Source: CAD feature listing. Evaluate the final solid. Frame: model axes, mm. A direction names the side the tool comes from. Round coordinates to 2 decimals unless told otherwise and drop trailing zeros. Write each loop counter-clockwise with the first axis right and the second up, starting at its lowest first coordinate (ties: lowest second). Pieces come first, ordered by that corner, then holes. Notation, with made-up numbers: M -28.75,-19.75 L 16.25,-19.75 A19 cw 16.25,-10.75 Z; hole C 75,-21 d3. An arc over 180 degrees is marked long. Answer in a Markdown table with one row per item.
from build123d import *

# Parameters (mm, degrees)
SKETCH1_W           = 2.4
SKETCH1_H           = 100
SKETCH1_W_2         = 92
SKETCH1_R           = 3
BOSS_EXTRUDE1_DEPTH = 5
SKETCH2_W           = 94.4
SKETCH2_H           = 7.5
BOSS_EXTRUDE2_DEPTH = 50
BOSS_EXTRUDE3_DEPTH = 5
LPATTERN1_COUNT     = 2
LPATTERN1_PITCH     = 27.6
LPATTERN1_COL_COUNT = 2
LPATTERN1_COL_PITCH = 27.6
FILLET1_R           = 3
CUT_EXTRUDE2_REACH  = 145.152
SKETCH9_R           = 1.7


with BuildPart() as part:
    # Sketch1 → Boss-Extrude1 (new body)
    # profile 1 of 2: a face of its own
    with BuildSketch(Plane.XY):
        with Locations((93.2, 50)):
            Rectangle(SKETCH1_W, SKETCH1_H)
    # profile 2 of 2: a face of its own
    with BuildSketch(Plane.XY):
        with Locations((46, 50)):
            Rectangle(SKETCH1_W_2, SKETCH1_H)
        with Locations((7.3, 20.94)):
            Circle(SKETCH1_R, mode=Mode.SUBTRACT)
        with Locations((87.1, 18.5)):
            Circle(SKETCH1_R, mode=Mode.SUBTRACT)
        with Locations((7.3, 66.66)):
            Circle(SKETCH1_R, mode=Mode.SUBTRACT)
        with Locations((87.1, 82.32)):
            Circle(SKETCH1_R, mode=Mode.SUBTRACT)
    extrude(amount=BOSS_EXTRUDE1_DEPTH)

    # Sketch2 → Boss-Extrude2 (add)
    with BuildSketch(Plane.XY.offset(5)):
        with Locations((47.2, 96.25)):
            Rectangle(SKETCH2_W, SKETCH2_H)
    extrude(amount=BOSS_EXTRUDE2_DEPTH)

    # Sketch7 → Boss-Extrude3 (add, symmetric)
    with BuildSketch(Plane(origin=(47.2, 0, 0), x_dir=(0, 0, -1), z_dir=(1, 0, 0))):
        Polygon((-55, 92.5), (-5, 0), (-5, 92.5), align=None)
    boss_extrude3 = extrude(amount=BOSS_EXTRUDE3_DEPTH, both=True)

    # LPattern1: Boss-Extrude3 ×2
    with Locations(*[(-i * LPATTERN1_PITCH, 0, 0) for i in range(1, LPATTERN1_COUNT)]):
        add(boss_extrude3)

    # LPattern1 col: Boss-Extrude3 ×2
    with Locations(*[(i * LPATTERN1_COL_PITCH, 0, 0) for i in range(1, LPATTERN1_COL_COUNT)]):
        add(boss_extrude3)

    # Fillet1
    fillet1_edges = [part.edges().sort_by_distance(p)[0] for p in [
        (47.2, 100, 0),
        (7.3, 92.5, 5),
        (61, 92.5, 5),
        (87.1, 92.5, 5),
        (33.4, 92.5, 5),
    ]]
    fillet(fillet1_edges, radius=FILLET1_R)

    # Sketch9 → Cut-Extrude2 (cut, up to next)
    with BuildSketch(Plane.XZ.offset(-92.5), mode=Mode.PRIVATE) as cut_extrude2_sk1:
        with Locations(Location((32.2, 50, 0), (0, 0, 270))):
            Circle(SKETCH9_R)
    cut_extrude2_tool1 = extrude(cut_extrude2_sk1.sketch, amount=-CUT_EXTRUDE2_REACH, mode=Mode.PRIVATE) & part.part
    # Sketch9 → Cut-Extrude2 (cut, up to next)
    with BuildSketch(Plane.XZ.offset(-92.5), mode=Mode.PRIVATE) as cut_extrude2_sk2:
        with Locations(Location((62.2, 50, 0), (0, 0, 270))):
            Circle(SKETCH9_R)
    cut_extrude2_tool2 = extrude(cut_extrude2_sk2.sketch, amount=-CUT_EXTRUDE2_REACH, mode=Mode.PRIVATE) & part.part
    # Sketch9 → Cut-Extrude2 (cut, up to next)
    with BuildSketch(Plane.XZ.offset(-92.5), mode=Mode.PRIVATE) as cut_extrude2_sk3:
        with Locations(Location((62.2, 40, 0), (0, 0, 270))):
            Circle(SKETCH9_R)
    cut_extrude2_tool3 = extrude(cut_extrude2_sk3.sketch, amount=-CUT_EXTRUDE2_REACH, mode=Mode.PRIVATE) & part.part
    # Sketch9 → Cut-Extrude2 (cut, up to next)
    with BuildSketch(Plane.XZ.offset(-92.5), mode=Mode.PRIVATE) as cut_extrude2_sk4:
        with Locations(Location((62.2, 30, 0), (0, 0, 270))):
            Circle(SKETCH9_R)
    cut_extrude2_tool4 = extrude(cut_extrude2_sk4.sketch, amount=-CUT_EXTRUDE2_REACH, mode=Mode.PRIVATE) & part.part
    # Sketch9 → Cut-Extrude2 (cut, up to next)
    with BuildSketch(Plane.XZ.offset(-92.5), mode=Mode.PRIVATE) as cut_extrude2_sk5:
        with Locations(Location((62.2, 20, 0), (0, 0, 270))):
            Circle(SKETCH9_R)
    cut_extrude2_tool5 = extrude(cut_extrude2_sk5.sketch, amount=-CUT_EXTRUDE2_REACH, mode=Mode.PRIVATE) & part.part
    # Sketch9 → Cut-Extrude2 (cut, up to next)
    with BuildSketch(Plane.XZ.offset(-92.5), mode=Mode.PRIVATE) as cut_extrude2_sk6:
        with Locations(Location((62.2, 10, 0), (0, 0, 270))):
            Circle(SKETCH9_R)
    cut_extrude2_tool6 = extrude(cut_extrude2_sk6.sketch, amount=-CUT_EXTRUDE2_REACH, mode=Mode.PRIVATE) & part.part
    # Sketch9 → Cut-Extrude2 (cut, up to next)
    with BuildSketch(Plane.XZ.offset(-92.5), mode=Mode.PRIVATE) as cut_extrude2_sk7:
        with Locations(Location((32.2, 40, 0), (0, 0, 270))):
            Circle(SKETCH9_R)
    cut_extrude2_tool7 = extrude(cut_extrude2_sk7.sketch, amount=-CUT_EXTRUDE2_REACH, mode=Mode.PRIVATE) & part.part
    # Sketch9 → Cut-Extrude2 (cut, up to next)
    with BuildSketch(Plane.XZ.offset(-92.5), mode=Mode.PRIVATE) as cut_extrude2_sk8:
        with Locations(Location((32.2, 30, 0), (0, 0, 270))):
            Circle(SKETCH9_R)
    cut_extrude2_tool8 = extrude(cut_extrude2_sk8.sketch, amount=-CUT_EXTRUDE2_REACH, mode=Mode.PRIVATE) & part.part
    # Sketch9 → Cut-Extrude2 (cut, up to next)
    with BuildSketch(Plane.XZ.offset(-92.5), mode=Mode.PRIVATE) as cut_extrude2_sk9:
        with Locations(Location((32.2, 20, 0), (0, 0, 270))):
            Circle(SKETCH9_R)
    cut_extrude2_tool9 = extrude(cut_extrude2_sk9.sketch, amount=-CUT_EXTRUDE2_REACH, mode=Mode.PRIVATE) & part.part
    # Sketch9 → Cut-Extrude2 (cut, up to next)
    with BuildSketch(Plane.XZ.offset(-92.5), mode=Mode.PRIVATE) as cut_extrude2_sk10:
        with Locations(Location((32.2, 10, 0), (0, 0, 270))):
            Circle(SKETCH9_R)
    cut_extrude2_tool10 = extrude(cut_extrude2_sk10.sketch, amount=-CUT_EXTRUDE2_REACH, mode=Mode.PRIVATE) & part.part
    add(cut_extrude2_tool1.solids().sort_by_distance((32.2, 92.5, 50))[0], mode=Mode.SUBTRACT)
    add(cut_extrude2_tool2.solids().sort_by_distance((62.2, 92.5, 50))[0], mode=Mode.SUBTRACT)
    add(cut_extrude2_tool3.solids().sort_by_distance((62.2, 92.5, 40))[0], mode=Mode.SUBTRACT)
    add(cut_extrude2_tool4.solids().sort_by_distance((62.2, 92.5, 30))[0], mode=Mode.SUBTRACT)
    add(cut_extrude2_tool5.solids().sort_by_distance((62.2, 92.5, 20))[0], mode=Mode.SUBTRACT)
    add(cut_extrude2_tool6.solids().sort_by_distance((62.2, 92.5, 10))[0], mode=Mode.SUBTRACT)
    add(cut_extrude2_tool7.solids().sort_by_distance((32.2, 92.5, 40))[0], mode=Mode.SUBTRACT)
    add(cut_extrude2_tool8.solids().sort_by_distance((32.2, 92.5, 30))[0], mode=Mode.SUBTRACT)
    add(cut_extrude2_tool9.solids().sort_by_distance((32.2, 92.5, 20))[0], mode=Mode.SUBTRACT)
    add(cut_extrude2_tool10.solids().sort_by_distance((32.2, 92.5, 10))[0], mode=Mode.SUBTRACT)


solid = part.part
Q1. Access query for faces 5 (the cylindrical face through (7.4, 91.64, 5.9)), 6 (the flat face through (47, 0, 2)), 7 (the cylindrical face through (33.52, 91.64, 5.9)). Directions: +Z, -Z, +X, -X, +Y, -Y. A direction counts if a zero-diameter tool reaches every point of the face in a straight line with its end or side. Return the directions, or none.
Solutions:
| item | result |
|---|---|
| face 5 | +Z, -X, -Y |
| face 6 | +Z, -Z, +X, -X, -Y |
| face 7 | +Z, -Y |
Q2. Pull-direction query (X, two-part tool) for faces 1 (the flat face through (47.27, 46.9, 30.35)), 2 (the flat face through (79.8, 67, 19)), 3 (the flat face through (14.6, 67, 19)), 4 (the cylindrical face through (89.87, 81.17, 2.46)); classes: pulls with the +X half, pulls with the -X half, needs draft (parallel to the pull), parting line crosses it, or undercut.
Solutions:
| item | result |
|---|---|
| face 1 | needs draft |
| face 2 | pulls with the +X half |
| face 3 | pulls with the -X half |
| face 4 | undercut |
Q3. Section A-A (z = 20). Return loops of the section in (x, y), and give its area (3 significant figures).
Solutions:
| item | result |
|---|---|
| outline | M 0,92.5 L 14.6,92.5 L 14.6,27.75 L 24.6,27.75 L 24.6,92.5 L 30.5,92.5 L 30.5,100 L 0,100 Z; M 33.9,92.5 L 42.2,92.5 L 42.2,27.75 L 52.2,27.75 L 52.2,92.5 L 60.5,92.5 L 60.5,100 L 33.9,100 Z; M 63.9,92.5 L 69.8,92.5 L 69.8,27.75 L 79.8,27.75 L 79.8,92.5 L 94.4,92.5 L 94.4,100 L 63.9,100 Z |
| area | 2,600 mm2 |
Q4. Section B-B (y = 82.32). Return loops of the section in (x, z), and give its area (3 significant figures).
Solutions:
| item | result |
|---|---|
| outline | M 0,0 L 84.1,0 L 84.1,5 L 79.8,5 L 79.8,49.5 L 69.8,49.5 L 69.8,5 L 52.2,5 L 52.2,49.5 L 42.2,49.5 L 42.2,5 L 24.6,5 L 24.6,49.5 L 14.6,49.5 L 14.6,5 L 0,5 Z; M 90.1,0 L 94.4,0 L 94.4,5 L 90.1,5 Z |
| area | 1,780 mm2 |
Q5. Contact query for flat-ended pins moving along their axis: pin 1 Ø8 at (x, z) = (32, 30) entering from +Y; pin 2 Ø5.5 at (x, z) = (58, 39.5) entering from -Y; pin 3 Ø12 at (y, z) = (68, 38) entering from -X; pin 4 Ø7.5 at (x, y) = (6.5, 45) entering from +Z. Output: stop coordinate, or through.
Solutions:
| item | result |
|---|---|
| pin 1 | stops at y = 100 |
| pin 2 | stops at y = 92.5 |
| pin 3 | stops at x = 14.6 |
| pin 4 | stops at z = 5 |
Q6. Section D-D (z = 34). Return loops of the section in (x, y), and give its area (3 significant figures).
Solutions:
| item | result |
|---|---|
| outline | M 0,92.5 L 14.6,92.5 L 14.6,53.65 L 24.6,53.65 L 24.6,92.5 L 42.2,92.5 L 42.2,53.65 L 52.2,53.65 L 52.2,92.5 L 69.8,92.5 L 69.8,53.65 L 79.8,53.65 L 79.8,92.5 L 94.4,92.5 L 94.4,100 L 0,100 Z |
| area | 1,870 mm2 |
Q7. Section C-C (x = 26). Return loops of the section in (y, z).
Solutions:
| item | result |
|---|---|
| outline | M 0,0 L 97,0 A3 ccw 100,3 L 100,55 L 92.5,55 L 92.5,8 A3 cw 89.5,5 L 0,5 Z |
Q8. Material intervals for probe 1 along X at (y, z) = (52, 6); probe 2 along X at (y, z) = (96.25, 50); probe 3 along Y at (x, z) = (34, 27), sorted ascending.
Solutions:
| item | result |
|---|---|
| probe 1 | x = 14.6 to 24.6, 42.2 to 52.2, 69.8 to 79.8 |
| probe 2 | x = 0 to 30.5, 33.9 to 60.5, 63.9 to 94.4 |
| probe 3 | y = 92.5 to 100 |
